from build123d import *
from OCP.BRepFilletAPI import BRepFilletAPI_MakeChamfer

# Parameters (mm, degrees)
SKETCH1_W                = 205
SKETCH1_H                = 130
BOSS_EXTRUDE1_DEPTH      = 10
SKETCH2_W                = 205
SKETCH2_H                = 130
SKETCH2_W_2              = 195
SKETCH2_H_2              = 120
BOSS_EXTRUDE2_DEPTH      = 40
CUT_EXTRUDE1_REACH       = 222.794
SKETCH6_W                = 60
SKETCH6_H                = 40
HOLE1_D                  = 4.8
HOLE1_DEPTH              = 8
HOLE1_CBORE_D            = 5.4
HOLE1_CBORE_DEPTH        = 6
CHAMFER1_SIZE            = 6
CHAMFER1_SIZE_2          = 0.3
BOSS_EXTRUDE3_DEPTH      = 15
FILLET1_R                = 5
HOLE2_D                  = 6.8
HOLE2_DEPTH              = 10
HOLE2_CBORE_D            = 7.4
HOLE2_CBORE_DEPTH        = 6
CHAMFER2_SIZE            = 6
CHAMFER2_SIZE_2          = 0.3
SKETCH14_W               = 179.585790587
SKETCH14_H               = 72.16534995
CUT_EXTRUDE2_DEPTH       = 150
SKETCH15_W               = 15.6
SKETCH15_H               = 3.6
SKETCH15_W_2             = 4.6
SKETCH15_H_2             = 7.6
BOSS_EXTRUDE4_DEPTH      = 12
M3_CLEARANCE_HOLE1_D     = 3.4
M3_CLEARANCE_HOLE1_DEPTH = 9.8


with BuildPart() as part:
    # Sketch1 → Boss-Extrude1 (new body)
    with BuildSketch(Plane(origin=(0, 0, 0), x_dir=(1, 0, 0), z_dir=(0, 1, 0))):
        Rectangle(SKETCH1_W, SKETCH1_H)
    extrude(amount=BOSS_EXTRUDE1_DEPTH)

    # Sketch2 → Boss-Extrude2 (add)
    with BuildSketch(Plane(origin=(0, 10, 0), x_dir=(1, 0, 0), z_dir=(0, 1, 0))):
        Rectangle(SKETCH2_W, SKETCH2_H)
        Rectangle(SKETCH2_W_2, SKETCH2_H_2, mode=Mode.SUBTRACT)
    extrude(amount=BOSS_EXTRUDE2_DEPTH)

    # Sketch6 → Cut-Extrude1 (cut, up to next)
    with BuildSketch(Plane.ZY.offset(102.5), mode=Mode.PRIVATE) as cut_extrude1_sk1:
        with Locations((-30, 30)):
            Rectangle(SKETCH6_W, SKETCH6_H)
    cut_extrude1_tool1 = extrude(cut_extrude1_sk1.sketch, amount=-CUT_EXTRUDE1_REACH, mode=Mode.PRIVATE) & part.part
    add(cut_extrude1_tool1.solids().sort_by_distance((-102.5, 30, -30))[0], mode=Mode.SUBTRACT)

    # Hole1
    with Locations(Plane(origin=(0, 10, 0), x_dir=(1, 0, 0), z_dir=(0, 1, 0))):
        with Locations((-84.35, -28.5), (-10.65, -28.5), (-78.5, 4.2), (-77.2, 52.4), (-26.4, 9.3), (-26.4, 37.2), (-2.3, 52.4), (4.05, 4.2), (29.2, 48.3), (65.8, 48.3), (65.8, 11.7), (29.2, 11.7), (10.65, -28.5), (84.35, -28.5)):
            CounterBoreHole(HOLE1_D / 2, HOLE1_CBORE_D / 2, HOLE1_CBORE_DEPTH, depth=HOLE1_DEPTH)

    # Chamfer1
    chamfer1_edges_1 = [part.edges().sort_by_distance(p)[0] for p in [
        (-5, 4, -52.4),
    ]]
    chamfer1_side_1 = [part.faces().sort_by_distance(p)[0] for p in [
        (-5, 4.006, -52.4),
    ]]
    chamfer1_edges_2 = [part.edges().sort_by_distance(p)[0] for p in [
        (-29.1, 4, -37.2),
    ]]
    chamfer1_side_2 = [part.faces().sort_by_distance(p)[0] for p in [
        (-29.1, 4.006, -37.2),
    ]]
    chamfer1_edges_3 = [part.edges().sort_by_distance(p)[0] for p in [
        (-29.1, 4, -9.3),
    ]]
    chamfer1_side_3 = [part.faces().sort_by_distance(p)[0] for p in [
        (-29.1, 4.006, -9.3),
    ]]
    chamfer1_edges_4 = [part.edges().sort_by_distance(p)[0] for p in [
        (-79.9, 4, -52.4),
    ]]
    chamfer1_side_4 = [part.faces().sort_by_distance(p)[0] for p in [
        (-79.9, 4.006, -52.4),
    ]]
    chamfer1_edges_5 = [part.edges().sort_by_distance(p)[0] for p in [
        (-81.2, 4, -4.2),
    ]]
    chamfer1_side_5 = [part.faces().sort_by_distance(p)[0] for p in [
        (-81.2, 4.006, -4.2),
    ]]
    chamfer1_edges_6 = [part.edges().sort_by_distance(p)[0] for p in [
        (-13.35, 4, 28.5),
    ]]
    chamfer1_side_6 = [part.faces().sort_by_distance(p)[0] for p in [
        (-13.35, 4.006, 28.5),
    ]]
    chamfer1_edges_7 = [part.edges().sort_by_distance(p)[0] for p in [
        (-87.05, 4, 28.5),
    ]]
    chamfer1_side_7 = [part.faces().sort_by_distance(p)[0] for p in [
        (-87.05, 4.006, 28.5),
    ]]
    chamfer1_edges_8 = [part.edges().sort_by_distance(p)[0] for p in [
        (81.65, 4, 28.5),
    ]]
    chamfer1_side_8 = [part.faces().sort_by_distance(p)[0] for p in [
        (81.65, 4.006, 28.5),
    ]]
    chamfer1_edges_9 = [part.edges().sort_by_distance(p)[0] for p in [
        (7.95, 4, 28.5),
    ]]
    chamfer1_side_9 = [part.faces().sort_by_distance(p)[0] for p in [
        (7.95, 4.006, 28.5),
    ]]
    chamfer1_edges_10 = [part.edges().sort_by_distance(p)[0] for p in [
        (26.5, 4, -11.7),
    ]]
    chamfer1_side_10 = [part.faces().sort_by_distance(p)[0] for p in [
        (26.5, 4.006, -11.7),
    ]]
    chamfer1_edges_11 = [part.edges().sort_by_distance(p)[0] for p in [
        (63.1, 4, -11.7),
    ]]
    chamfer1_side_11 = [part.faces().sort_by_distance(p)[0] for p in [
        (63.1, 4.006, -11.7),
    ]]
    chamfer1_edges_12 = [part.edges().sort_by_distance(p)[0] for p in [
        (63.1, 4, -48.3),
    ]]
    chamfer1_side_12 = [part.faces().sort_by_distance(p)[0] for p in [
        (63.1, 4.006, -48.3),
    ]]
    chamfer1_edges_13 = [part.edges().sort_by_distance(p)[0] for p in [
        (26.5, 4, -48.3),
    ]]
    chamfer1_side_13 = [part.faces().sort_by_distance(p)[0] for p in [
        (26.5, 4.006, -48.3),
    ]]
    chamfer1_edges_14 = [part.edges().sort_by_distance(p)[0] for p in [
        (1.35, 4, -4.2),
    ]]
    chamfer1_side_14 = [part.faces().sort_by_distance(p)[0] for p in [
        (1.35, 4.006, -4.2),
    ]]
    chamfer1 = BRepFilletAPI_MakeChamfer(part.part.solid().wrapped)
    for e in chamfer1_edges_1:
        chamfer1.Add(CHAMFER1_SIZE - 0.0001, CHAMFER1_SIZE_2 - 0.0001, e.wrapped, chamfer1_side_1[0].wrapped)
    for e in chamfer1_edges_2:
        chamfer1.Add(CHAMFER1_SIZE - 0.0001, CHAMFER1_SIZE_2 - 0.0001, e.wrapped, chamfer1_side_2[0].wrapped)
    for e in chamfer1_edges_3:
        chamfer1.Add(CHAMFER1_SIZE - 0.0001, CHAMFER1_SIZE_2 - 0.0001, e.wrapped, chamfer1_side_3[0].wrapped)
    for e in chamfer1_edges_4:
        chamfer1.Add(CHAMFER1_SIZE - 0.0001, CHAMFER1_SIZE_2 - 0.0001, e.wrapped, chamfer1_side_4[0].wrapped)
    for e in chamfer1_edges_5:
        chamfer1.Add(CHAMFER1_SIZE - 0.0001, CHAMFER1_SIZE_2 - 0.0001, e.wrapped, chamfer1_side_5[0].wrapped)
    for e in chamfer1_edges_6:
        chamfer1.Add(CHAMFER1_SIZE - 0.0001, CHAMFER1_SIZE_2 - 0.0001, e.wrapped, chamfer1_side_6[0].wrapped)
    for e in chamfer1_edges_7:
        chamfer1.Add(CHAMFER1_SIZE - 0.0001, CHAMFER1_SIZE_2 - 0.0001, e.wrapped, chamfer1_side_7[0].wrapped)
    for e in chamfer1_edges_8:
        chamfer1.Add(CHAMFER1_SIZE - 0.0001, CHAMFER1_SIZE_2 - 0.0001, e.wrapped, chamfer1_side_8[0].wrapped)
    for e in chamfer1_edges_9:
        chamfer1.Add(CHAMFER1_SIZE - 0.0001, CHAMFER1_SIZE_2 - 0.0001, e.wrapped, chamfer1_side_9[0].wrapped)
    for e in chamfer1_edges_10:
        chamfer1.Add(CHAMFER1_SIZE - 0.0001, CHAMFER1_SIZE_2 - 0.0001, e.wrapped, chamfer1_side_10[0].wrapped)
    for e in chamfer1_edges_11:
        chamfer1.Add(CHAMFER1_SIZE - 0.0001, CHAMFER1_SIZE_2 - 0.0001, e.wrapped, chamfer1_side_11[0].wrapped)
    for e in chamfer1_edges_12:
        chamfer1.Add(CHAMFER1_SIZE - 0.0001, CHAMFER1_SIZE_2 - 0.0001, e.wrapped, chamfer1_side_12[0].wrapped)
    for e in chamfer1_edges_13:
        chamfer1.Add(CHAMFER1_SIZE - 0.0001, CHAMFER1_SIZE_2 - 0.0001, e.wrapped, chamfer1_side_13[0].wrapped)
    for e in chamfer1_edges_14:
        chamfer1.Add(CHAMFER1_SIZE - 0.0001, CHAMFER1_SIZE_2 - 0.0001, e.wrapped, chamfer1_side_14[0].wrapped)
    add(Compound.cast(chamfer1.Shape()), mode=Mode.REPLACE)  # a hair under: the kernel refuses the full size

    # Sketch11 → Boss-Extrude3 (add)
    with BuildSketch(Plane(origin=(0, 50, 0), x_dir=(1, 0, 0), z_dir=(0, 1, 0))):
        Polygon((-112.5, 75), (112.5, 75), (112.5, -75), (-112.5, -75), (-112.5, 0), (-102.5, 0), (-102.5, -65), (102.5, -65), (102.5, 65), (-102.5, 65), (-102.5, 60), (-112.5, 60), align=None)
    extrude(amount=-BOSS_EXTRUDE3_DEPTH)

    # Fillet1
    fillet1_edges = [part.edges().sort_by_distance(p)[0] for p in [
        (-112.5, 35, 37.5),
        (0, 35, 75),
        (112.5, 35, 0),
        (0, 35, -75),
        (-102.5, 35, -62.5),
        (0, 35, -65),
        (102.5, 35, 0),
        (-102.5, 35, 32.5),
        (0, 35, 65),
    ]]
    fillet(fillet1_edges, radius=FILLET1_R - 0.0001)  # a hair under: the kernel refuses the full size

    # Hole2
    with Locations(Plane(origin=(0, 50, 0), x_dir=(1, 0, 0), z_dir=(0, 1, 0))):
        with Locations((-105, 67.5), (105, 67.5), (105, -67.5), (-105, -67.5)):
            CounterBoreHole(HOLE2_D / 2, HOLE2_CBORE_D / 2, HOLE2_CBORE_DEPTH, depth=HOLE2_DEPTH)

    # Chamfer2
    chamfer2_edges_1 = [part.edges().sort_by_distance(p)[0] for p in [
        (-108.7, 44, 67.5),
    ]]
    chamfer2_side_1 = [part.faces().sort_by_distance(p)[0] for p in [
        (-108.7, 44.006, 67.5),
    ]]
    chamfer2_edges_2 = [part.edges().sort_by_distance(p)[0] for p in [
        (101.3, 44, 67.5),
    ]]
    chamfer2_side_2 = [part.faces().sort_by_distance(p)[0] for p in [
        (101.3, 44.006, 67.5),
    ]]
    chamfer2_edges_3 = [part.edges().sort_by_distance(p)[0] for p in [
        (101.3, 44, -67.5),
    ]]
    chamfer2_side_3 = [part.faces().sort_by_distance(p)[0] for p in [
        (101.3, 44.006, -67.5),
    ]]
    chamfer2_edges_4 = [part.edges().sort_by_distance(p)[0] for p in [
        (-108.7, 44, -67.5),
    ]]
    chamfer2_side_4 = [part.faces().sort_by_distance(p)[0] for p in [
        (-108.7, 44.006, -67.5),
    ]]
    chamfer2 = BRepFilletAPI_MakeChamfer(part.part.solid().wrapped)
    for e in chamfer2_edges_1:
        chamfer2.Add(CHAMFER2_SIZE - 0.0001, CHAMFER2_SIZE_2 - 0.0001, e.wrapped, chamfer2_side_1[0].wrapped)
    for e in chamfer2_edges_2:
        chamfer2.Add(CHAMFER2_SIZE - 0.0001, CHAMFER2_SIZE_2 - 0.0001, e.wrapped, chamfer2_side_2[0].wrapped)
    for e in chamfer2_edges_3:
        chamfer2.Add(CHAMFER2_SIZE - 0.0001, CHAMFER2_SIZE_2 - 0.0001, e.wrapped, chamfer2_side_3[0].wrapped)
    for e in chamfer2_edges_4:
        chamfer2.Add(CHAMFER2_SIZE - 0.0001, CHAMFER2_SIZE_2 - 0.0001, e.wrapped, chamfer2_side_4[0].wrapped)
    add(Compound.cast(chamfer2.Shape()), mode=Mode.REPLACE)  # a hair under: the kernel refuses the full size

    # Sketch14 → Cut-Extrude2 (cut)
    with BuildSketch(Plane.ZY.offset(17.5)):
        with Locations((-1.737927005, 26.484477579)):
            Rectangle(SKETCH14_W, SKETCH14_H)
    extrude(amount=CUT_EXTRUDE2_DEPTH, mode=Mode.SUBTRACT)

    # Sketch15 → Boss-Extrude4 (add)
    with BuildSketch(Plane.ZY.offset(17.5)):
        with Locations((-51, 5)):
            Rectangle(SKETCH15_W, SKETCH15_H)
        with Locations((51, 5)):
            Rectangle(SKETCH15_W, SKETCH15_H)
        with Locations((0, 5)):
            Rectangle(SKETCH15_W, SKETCH15_H)
        with Locations((-67.5, 43)):
            Rectangle(SKETCH15_W_2, SKETCH15_H_2)
        with Locations((67.5, 43)):
            Rectangle(SKETCH15_W_2, SKETCH15_H_2)
    extrude(amount=BOSS_EXTRUDE4_DEPTH)

    # M3 Clearance Hole1
    with Locations(Plane.XY.offset(-65.2)):
        with Locations((-23.5, 43)):
            m3_clearance_hole1 = Hole(M3_CLEARANCE_HOLE1_D / 2, depth=M3_CLEARANCE_HOLE1_DEPTH)

    # Mirror1: M3 Clearance Hole1 across plane
    add(m3_clearance_hole1.mirror(Plane.XY), mode=Mode.SUBTRACT)


solid = part.part
Build history of the part. All positions in model axes, mm. A direction names the side the tool comes from. Give positions to 0.01 mm unless a question says otherwise; leave off trailing zeros. Order: outer loops, then holes, each group sorted by start corner. A loop starts at its lowest first (then second) coordinate and runs counter-clockwise, first axis right, second up. Notation, with made-up numbers: M 15,-37 L 39,-37 A16 cw 39,-27 Z; hole C -4,40 d2. An arc over 180 degrees is marked long. Use one line per item in the form item = value.
1) Tool access for faces 1 (the face through (-23, 5, 43.2)), 2 (the face through (107.698, 41.972, -65.431)), 3 (the face through (-23, 3.2, -51)): list every direction of +Z, -Z, +X, -X, +Y, -Y with a clear straight run to the whole face (end or side of a thin tool).
Calculated:
face_1 = -X, +Y, -Y
face_2 = +Y
face_3 = +Z, -Z, -X, -Y
2) Probe probe 1 along X at (y, z) = (3, -48); probe 2 along Z at (x, y) = (105, 42.5); probe 3 along Z at (x, y) = (79, 25). List the from-to ranges inside material, lowest first.
Calculated:
probe_1 = -17.5 to 26.82, 31.58 to 63.42, 68.18 to 102.5
probe_2 = -75 to -70.9, -64.1 to 64.1, 70.9 to 75
probe_3 = -65 to -60, 60 to 65
3) Two-plate mould, pull along Z, no slides. Class faces 4 (the face through (-29.5, 43, -68)), 5 (the face through (68.23, 6.96, -12.47)), 6 (the face through (-23, 41, 69.8)): released by +Z, released by -Z, zero draft, split by the parting line, or undercut.
Calculated:
face_4 = zero draft
face_5 = undercut
face_6 = released by +Z
4) Drop flat-ended pins along their axis: pin 1 (9 mm diameter, centred on x = 105, z = 67.5, fed in from +Y); pin 2 (2 mm diameter, centred on x = 28, z = 51, fed in from +Y); pin 3 (6 mm diameter, centred on y = 35.5, z = 3, fed in from +X); pin 4 (3.5 mm diameter, centred on x = -20.5, z = -66.5, fed in from +Y). Give the stop position or say it passes through.
Calculated:
pin_1 = 50
pin_2 = 10
pin_3 = 112.27
pin_4 = 46.8
5) Saw through at C-C (y = 20). Give the cut face in (x, z).
Calculated:
outline = M -17.5,-65 L 102.5,-65 L 102.5,65 L -17.5,65 L -17.5,60 L 97.5,60 L 97.5,-60 L -17.5,-60 Z
